Check sheet for the modelled part. Datum: model origin and axes. Units: mm. A direction names the side the tool comes from. Round coordinates to 2 decimals unless told otherwise and drop trailing zeros. Write each loop counter-clockwise with the first axis right and the second up, starting at its lowest first coordinate (ties: lowest second). Pieces come first, ordered by that corner, then holes.
Item 1: Tool access check on faces 4 (the flat face through (-30, 1, 4)), 5 (the flat face through (30, 1, 4)), 6 (the flat face through (-36, 1, 0)), 7 (the flat face through (-30, 1, -4)). Record the directions out of +Z, -Z, +X, -X, +Y, -Y that give a thin tool (end or side, any length) a straight path to the whole face; none if there is none.
Item 2: Cross-section at D-D on y = 5.25. Enter the section's corners in (x, z), plus the area to 3 significant figures.
Item 3: Material ranges on line 1 (Z direction, x = 0, y = 3.25); line 2 (X direction, y = 2.5, z = 1), recorded low to high.
Item 4: Go/stop test with flat-tipped pins: pin 1 Ø3.5 at (x, y) = (-29, 1) entering from -Z; pin 2 Ø2.5 at (x, z) = (-31, 1) entering from +Y; pin 3 Ø1.5 at (y, z) = (7, -5) entering from +X. Record where each tip stops, or that it passes through.
Item 5: Release check for a two-part mould opening along X. For faces 1 (the cylindrical face through (35.4, 1.48, -3.43)), 2 (the cylindrical face through (-30.215, 1.479, -0.234)), 3 (the flat face through (30, 1, -4)) record: +X half, -X half, draft (parallel to the pull), parting line (faces both ways), or undercut.
Item 6: Cross-section at C-C on z = 5.5. Enter the section's corners in (x, y), plus the area to 3 significant figures.
Item 7: Cross-section at A-A on x = -32. Enter the section's corners in (y, z), plus the area to 3 significant figures.
Item 8: Cross-section at B-B on z = 0. Enter the section's corners in (x, y).
from build123d import *

# Parameters (mm, degrees)
SKETCH1_R           = 27
SKETCH1_R_2         = 24
BOSS_EXTRUDE1_DEPTH = 10
SKETCH3_R           = 1.8
BOSS_EXTRUDE2_DEPTH = 3


with BuildPart() as part:
    # Sketch1 → Boss-Extrude1 (new body)
    with BuildSketch(Plane(origin=(0, 0, 0), x_dir=(1, 0, 0), z_dir=(0, 1, 0))):
        with Locations(Location((0, 0, 0), (0, 0, 270))):
            Circle(SKETCH1_R)
        with Locations(Location((0, 0, 0), (0, 0, 270))):
            Circle(SKETCH1_R_2, mode=Mode.SUBTRACT)
    extrude(amount=BOSS_EXTRUDE1_DEPTH)

    # Sketch3 → Boss-Extrude2 (add)
    with BuildSketch(Plane(origin=(0, 0, 0), x_dir=(1, 0, 0), z_dir=(0, 1, 0))):
        with BuildLine():
            Line((-24, 0), (-24, 4))
            Line((-24, 4), (-34, 4))
            ThreePointArc((-34, 4), (-35.414213562, 3.414213562), (-36, 2))
            Line((-36, 2), (-36, -2))
            ThreePointArc((-36, -2), (-35.414213562, -3.414213562), (-34, -4))
            Line((-34, -4), (-24, -4))
            Line((-24, -4), (-24, 0))
        make_face()
        with Locations(Location((-32, 0, 0), (0, 0, 270))):
            Circle(SKETCH3_R, mode=Mode.SUBTRACT)
    boss_extrude2 = extrude(amount=BOSS_EXTRUDE2_DEPTH)

    # Mirror1: Boss-Extrude2 across plane
    add(boss_extrude2.mirror(Plane(origin=(0, 0, 0), x_dir=(0, 0, 1), z_dir=(1, 0, 0))))


solid = part.part
Response values:
1. face 4: +Z, -X, +Y, -Y
1. face 5: +Z, +X, +Y, -Y
1. face 6: +Z, -Z, -X, +Y, -Y
1. face 7: -Z, -X, +Y, -Y
2. outline: circle Ø54 at (0, 0); hole circle Ø48 at (0, 0)
2. area: 481 mm2
3. line 1: z = -27 to -24, 24 to 27
3. line 2: x = -36 to -33.5, -30.5 to -23.98, 23.98 to 30.5, 33.5 to 36
4. pin 1: stops at z = -4
4. pin 2: stops at y = 3
4. pin 3: stops at x = 26.66
5. face 1: +X half
5. face 2: undercut
5. face 3: draft
6. outline: (-26.43, 0) - (-23.36, 0) - (-23.36, 10) - (-26.43, 10) - close; (23.36, 0) - (26.43, 0) - (26.43, 10) - (23.36, 10) - close
6. area: 61.5 mm2
7. outline: (0, -4) - (3, -4) - (3, -1.8) - (0, -1.8) - close; (0, 1.8) - (3, 1.8) - (3, 4) - (0, 4) - close
7. area: 13.2 mm2
8. outline: (-36, 0) - (-33.8, 0) - (-33.8, 3) - (-36, 3) - close; (-30.2, 0) - (-24, 0) - (-24, 10) - (-27, 10) - (-27, 3) - (-30.2, 3) - close; (24, 0) - (30.2, 0) - (30.2, 3) - (27, 3) - (27, 10) - (24, 10) - close; (33.8, 0) - (36, 0) - (36, 3) - (33.8, 3) - close
